Source: CAD feature listing. Evaluate the final solid. Frame: model axes, mm. A direction names the side the tool comes from. Give positions to 0.01 mm unless a question says otherwise; leave off trailing zeros. Order: outer loops, then holes, each group sorted by start corner. A loop starts at its lowest first (then second) coordinate and runs counter-clockwise, first axis right, second up. Notation, with made-up numbers: (-1, -1.75) - (22, -1.75) arc R10 cw to (22, 10.25) - close; hole circle Ø9 at (73, 51). An arc over 180 degrees is marked (long way). Use CSV: the item, a comma, the result in double quotes.
```python
from build123d import *

# Parameters (mm, degrees)
F0_W     = 40
F0_H     = 30
F1_DEPTH = 20
F2_R     = 1.75
F3_DEPTH = 40.001
F4_R     = 2
F5_DEPTH = 4
F6_R     = 0.5
F7_DEPTH = 16.001


with BuildPart() as f1:
    # F0 (on Top) → F1 (new body)
    with BuildSketch(Plane.XY):
        Rectangle(F0_W, F0_H)
    extrude(amount=F1_DEPTH)

    # F2 (on face) → F3 (cut, through all)
    with BuildSketch(Plane(origin=(-20, 0, 0), x_dir=(0, -1, 0), z_dir=(-1, 0, 0))):
        with Locations((-7.5, 10)):
            Circle(F2_R)
        with Locations((7.5, 10)):
            Circle(F2_R)
    extrude(amount=-F3_DEPTH, mode=Mode.SUBTRACT)

    # F4 (on face) → F5 (cut)
    with BuildSketch(Plane.XY.offset(20)):
        with Locations((15, 7.5)):
            Circle(F4_R)
        with Locations((-15, -7.5)):
            Circle(F4_R)
    extrude(amount=-F5_DEPTH, mode=Mode.SUBTRACT)

    # F6 (on face) → F7 (cut, through all)
    with BuildSketch(Plane.XY.offset(16)):
        with Locations((15, 7.5)):
            Circle(F6_R)
        with Locations((-15, -7.5)):
            Circle(F6_R)
    extrude(amount=-F7_DEPTH, mode=Mode.SUBTRACT)


solid = f1.part
```
Item 1: Section A-A on z = 10. Return the cut outline in (x, y), then the cut area to 3 significant figures.
Filled in:
outline,"(-20, -15) - (20, -15) - (20, -9.25) - (-20, -9.25) - close; (-20, -5.75) - (20, -5.75) - (20, 5.75) - (-20, 5.75) - close; (-20, 9.25) - (20, 9.25) - (20, 15) - (-20, 15) - close"
area,"920 mm2"
Item 2: Material intervals for line 1 (Y direction, x = -15, z = 18.8); line 2 (X direction, y = 7.5, z = 14.05); line 3 (Z direction, x = 0.5, y = -7.5), sorted ascending. Write a range as from..to.
Filled in:
line 1,"y = -15..-9.5, -5.5..15"
line 2,"x = -20..14.5, 15.5..20"
line 3,"z = 0..8.25, 11.75..20"
Item 3: First-contact query: pin 1 (1.2 mm diameter, centred on x = -16, y = -7, fed in from +Z). Flat tip, straight axial feed; report the tip coordinate or a pass-through.
Filled in:
pin 1,"stops at z = 16"
Item 4: Mould query, pull axis Y, two halves, no side actions, for faces 3 (the flat face through (0, 15, 10)), 4 (the cylindrical face through (-15, -8, 4)), 5 (the flat face through (20, 0, 10)), 6 (the flat face through (0, -15, 10)). Classes: released by +Y, released by -Y, zero draft, split by the parting line, or undercut.
Filled in:
face 3,"released by +Y"
face 4,"undercut"
face 5,"zero draft"
face 6,"released by -Y"
Item 5: Section D-D on x = 10.5. Return the cut outline in (y, z).
Filled in:
outline,"(-15, 0) - (15, 0) - (15, 20) - (-15, 20) - close; hole circle Ø3.5 at (-7.5, 10); hole circle Ø3.5 at (7.5, 10)"
Item 6: Section C-C on x = 15. Return the cut outline in (y, z), then the cut area to 3 significant figures.
Filled in:
outline,"(-15, 0) - (7, 0) - (7, 8.32) arc R1.75 cw to (7, 11.68) - (7, 16) - (5.5, 16) - (5.5, 20) - (-15, 20) - close; (8, 0) - (15, 0) - (15, 20) - (9.5, 20) - (9.5, 16) - (8, 16) - (8, 11.68) arc R1.75 cw to (8, 8.32) - close; hole circle Ø3.5 at (-7.5, 10)"
area,"552 mm2"
Item 7: Set-up query: faces 1 (the flat face through (0, 0, 0)), 2 (the cylindrical face through (13.526, 8.852, 18.028)). Return all of +Z, -Z, +X, -X, +Y, -Y with unobstructed straight access to the full face (end or side cutting, diameter ignored); none if empty.
Filled in:
face 1,"-Z, +X, -X, +Y, -Y"
face 2,"+Z"
Item 8: Section B-B on y = 7.5. Return the cut outline in (x, z).
Filled in:
outline,"(-20, 0) - (14.5, 0) - (14.5, 8.25) - (-20, 8.25) - close; (-20, 11.75) - (14.5, 11.75) - (14.5, 16) - (13, 16) - (13, 20) - (-20, 20) - close; (15.5, 0) - (20, 0) - (20, 8.25) - (15.5, 8.25) - close; (15.5, 11.75) - (20, 11.75) - (20, 20) - (17, 20) - (17, 16) - (15.5, 16) - close"
